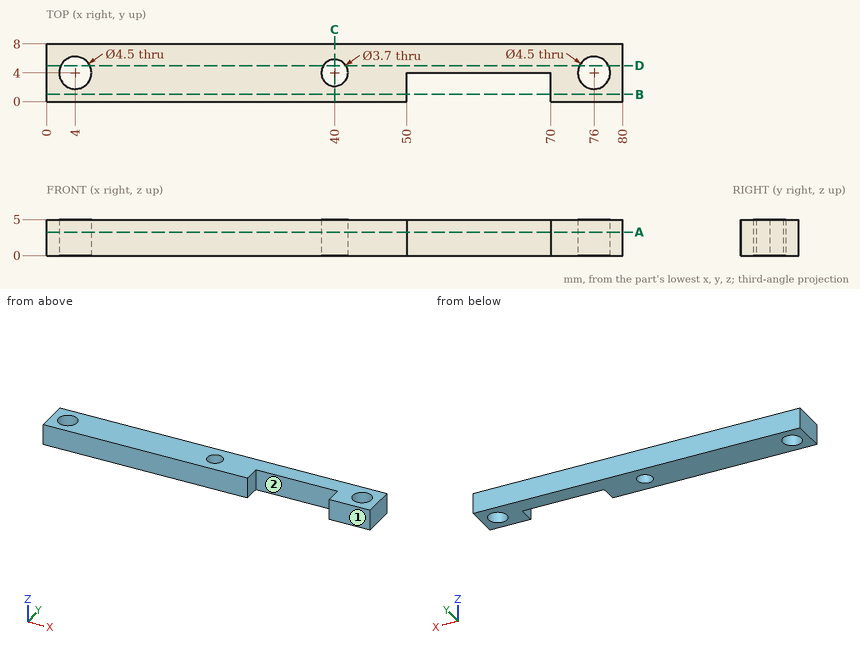
Can you work these out from the drawing? Everything is in mm from the part's minimum corner. Give positions to 0.01 mm unless a question says otherwise; leave off trailing zeros. Order: outer loops, then holes, each group sorted by start corner. A loop starts at its lowest first (then second) coordinate and runs counter-clockwise, first axis right, second up. Notation, with made-up numbers: M 85.5,76.5 L 115.5,76.5 A27 cw 115.5,110.5 Z; hole C 37,53.5 d3. An arc over 180 degrees is marked long. Use a Markdown table: item, result. Add a question column.
Item 1: We'd pull the mould along X, two halves only. Please class the marked faces 1 and 2: +X half, -X half, draft (parallel to the pull), parting line (faces both ways), or undercut.
Item 2: Suppose I cut it at C-C (x = 40). List the corners of the cut face in (y, z) for me, then the cut area to 3 significant figures.
Item 3: Will this pin go through, and if not, where does the flat tip stop? pin 1 (2.5 mm diameter, centred on x = 61, z = 2, fed in from -Y).
Item 4: Suppose I cut it at D-D (y = 5). List the corners of the cut face in (x, z) for me.
Item 5: Suppose I cut it at B-B (y = 1). List the corners of the cut face in (x, z) for me.
Item 6: If I drill on L1, parallel to Y at x = 76, z = 3.25; L2, parallel to Y at x = 40, z = 2.2; L3, parallel to X at y = 5.25, z = 1.05, over which ranges is the centre line in solid material (lowest first)? Write a range as [from, to].
Item 7: Suppose I cut it at A-A (z = 3.25). List the corners of the cut face in (x, y) for me.
Answer sheet:
| question | item | result |
|---|---|---|
| 1 | face 1 | draft |
| 1 | face 2 | undercut |
| 2 | outline | M 0,0 L 2.15,0 L 2.15,5 L 0,5 Z; M 5.85,0 L 8,0 L 8,5 L 5.85,5 Z |
| 2 | area | 21.5 mm² |
| 3 | pin 1 | stops at y = 4 |
| 4 | outline | M 0,0 L 1.98,0 L 1.98,5 L 0,5 Z; M 6.02,0 L 38.44,0 L 38.44,5 L 6.02,5 Z; M 41.56,0 L 73.98,0 L 73.98,5 L 41.56,5 Z; M 78.02,0 L 80,0 L 80,5 L 78.02,5 Z |
| 5 | outline | M 0,0 L 50,0 L 50,5 L 0,5 Z; M 70,0 L 80,0 L 80,5 L 70,5 Z |
| 6 | L1 | y = [0, 1.75], [6.25, 8] |
| 6 | L2 | y = [0, 2.15], [5.85, 8] |
| 6 | L3 | x = [0, 2.13], [5.87, 38.64], [41.36, 74.13], [77.87, 80] |
| 7 | outline | M 0,0 L 50,0 L 50,4 L 70,4 L 70,0 L 80,0 L 80,8 L 0,8 Z; hole C 4,4 d4.5; hole C 40,4 d3.7; hole C 76,4 d4.5 |
